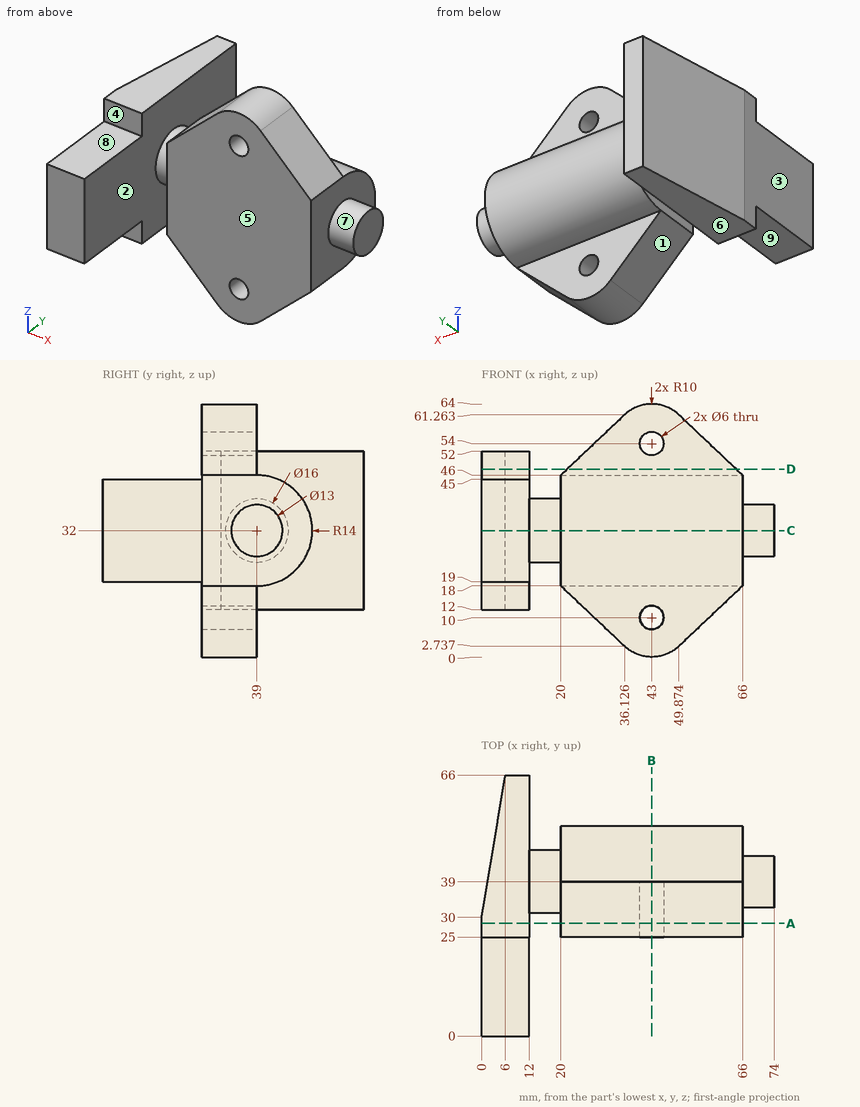
Check sheet for the drawn part. Datum: minimum x, y, z corner. Units: mm. A direction names the side the tool comes from. Coordinates: 2 decimals unless noted, no trailing zeros. Write each loop counter-clockwise with the first axis right and the second up, starting at its lowest first coordinate (ties: lowest second). Pieces come first, ordered by that corner, then holes. Notation, with made-up numbers: (18, 66) - (48, 66) arc R29 cw to (48, 101) - close; hole circle Ø2 at (-15.75, 74.5). An arc over 180 degrees is marked (long way). Answer as a JSON object with one key per item and string values.
(1) Cross-section at D-D on z = 47.5. Record the cut outline in (x, y) (1 decimal), plus the area to 3 significant figures.
Report:
{"outline": "(0, 25) - (12, 25) - (12, 66) - (6, 66) - (0, 30) - close; (21.6, 25) - (64.4, 25) - (64.4, 39) - (21.6, 39) - close", "area": "984 mm^2"}
(2) Cross-section at B-B on x = 43. Record the cut outline in (y, z), plus the area to 3 significant figures.
Report:
{"outline": "(25, 0) - (39, 0) - (39, 7) - (25, 7) - close; (25, 13) - (39, 13) - (39, 18) arc R14 ccw to (39, 46) - (39, 51) - (25, 51) - close; (25, 57) - (39, 57) - (39, 64) - (25, 64) - close", "area": "1,040 mm^2"}
(3) Tool access check on the marked faces 5, 6, 7, 8 and 9. Record the directions out of +Z, -Z, +X, -X, +Y, -Y that give a thin tool (end or side, any length) a straight path to the whole face; none if there is none.
Report:
{"face 5": "+Z, -Z, +X, -Y", "face 6": "-Z, -X, +Y, -Y", "face 7": "+X", "face 8": "+Z, +X, -X, -Y", "face 9": "-Z, +X, -X, -Y"}
(4) Cross-section at C-C on z = 32. Record the cut outline in (x, y), plus the area to 3 significant figures.
Report:
{"outline": "(0, 0) - (12, 0) - (12, 31) - (20, 31) - (20, 25) - (66, 25) - (66, 32.5) - (74, 32.5) - (74, 45.5) - (66, 45.5) - (66, 53) - (20, 53) - (20, 47) - (12, 47) - (12, 66) - (6, 66) - (0, 30) - close", "area": "2,200 mm^2"}
(5) Thickness scan on line 1 along Z through (x, y) = (43, 28.5); line 2 along X through (y, z) = (13.5, 24); line 3 along Y through (x, z) = (26.5, 52). Record the ranges inside material, lowest first.
Report:
{"line 1": "0 to 7, 13 to 51, 57 to 64", "line 2": "0 to 12", "line 3": "25 to 39"}
(6) Gauge pin test, flat ends, axial feed: pin 1 Ø3.5 at (x, y) = (7, 43.5) entering from -Z; pin 2 Ø14.5 at (x, z) = (46, 55.5) entering from +Y; pin 3 Ø6 at (x, y) = (6, 16.5) entering from +Z. Record the tip position at first contact, or that the pin passes through.
Report:
{"pin 1": "z = 12", "pin 2": "y = 39", "pin 3": "z = 45"}
(7) Mould release check, pull along X, two halves, no side actions. Record for the marked faces 1, 2, 3 and 4: pulls with the +X half, pulls with the -X half, needs draft (parallel to the pull), parting line crosses it, or undercut.
Report:
{"face 1": "undercut", "face 2": "undercut", "face 3": "pulls with the -X half", "face 4": "needs draft"}
(8) Cross-section at A-A on y = 28.5. Record the cut outline in (x, z), plus the area to 4 significant figures.
Report:
{"outline": "(0, 12) - (12, 12) - (12, 52) - (0, 52) - close; (20, 18) - (36.13, 2.74) arc R10 ccw to (49.87, 2.74) - (66, 18) - (66, 46) - (49.87, 61.26) arc R10 ccw to (36.13, 61.26) - (20, 46) - close; hole circle Ø6 at (43, 10); hole circle Ø6 at (43, 54)", "area": "2,675 mm^2"}
